from build123d import *

# Parameters (mm, degrees)
F0_R         = 5
F1_DEPTH     = 66
F2_R         = 5
F3_DEPTH     = 25
F5_DEPTH     = 11
F6_T1_DEPTH  = 14.0560753695
F6_T3_DEPTH  = 14.0560753695
F6_T5_DEPTH  = 14.0560753695
F6_T7_DEPTH  = 14.0560753695
F6_T9_DEPTH  = 14.0560753695
F6_T11_DEPTH = 14.0560753695
F6_T13_DEPTH = 17.3577997637
F6_T15_DEPTH = 17.3577997637
F6_T18_ANGLE = 298.0668340959


# Not quite as in the source:
# - a fillet or chamfer that OpenCascade refuses, or shapes differently, is made with other operations: its cross-section is extruded or revolved along the edge and cut away or added


with BuildPart() as f1:
    # F0 (on Top) → F1 (new body)
    with BuildSketch(Plane.XY):
        Circle(F0_R)
    extrude(amount=F1_DEPTH)

    # F2 (on face) → F3 (cut)
    with BuildSketch(Plane.XY.offset(66)):
        Circle(F2_R)
        Polygon((4.55, 1.8846717088), (4.55, -1.8846717088), (1.8846717088, -4.55), (-1.8846717088, -4.55), (-4.55, -1.8846717088), (-4.55, 1.8846717088), (-1.8846717088, 4.55), (1.8846717088, 4.55), align=None, mode=Mode.SUBTRACT)
    extrude(amount=-F3_DEPTH, mode=Mode.SUBTRACT)

    # F4 (on face) → F5 (cut)
    with BuildSketch(Plane(origin=(0, 0, 0), x_dir=(1, 0, 0), z_dir=(0, 0, -1))):
        with BuildLine():
            ThreePointArc((5, 0), (4.6193976626, 1.9134171618), (3.5355339059, 3.5355339059))
            Line((3.5355339059, 3.5355339059), (3.5355339059, -3.5355339059))
            ThreePointArc((3.5355339059, -3.5355339059), (4.6193976626, -1.9134171618), (5, 0))
        make_face()
        with BuildLine():
            ThreePointArc((-3.5355339059, -3.5355339059), (0, -5), (3.5355339059, -3.5355339059))
            Line((3.5355339059, -3.5355339059), (-3.5355339059, -3.5355339059))
        make_face()
    extrude(amount=-F5_DEPTH, mode=Mode.SUBTRACT)

    # F6: chamfer of 2 on 11 edges, made by hand

    # F6_s2 → F6_t1 (cut)
    with BuildSketch(Plane(origin=(-4.9695731053, 4.9695731053, 0), x_dir=(0, 0, 1), z_dir=(0.7071067812, -0.7071067812, 0))):
        Polygon((64, -4.55), (66, -2.55), (66, -4.55), align=None)
    extrude(amount=F6_T1_DEPTH, mode=Mode.SUBTRACT)

    # F6_s4 → F6_t3 (cut)
    with BuildSketch(Plane.XZ.offset(-7.0280376847)):
        Polygon((4.55, 64), (2.55, 66), (4.55, 66), align=None)
        Polygon((-4.55, 64), (-2.55, 66), (-4.55, 66), align=None)
    extrude(amount=F6_T3_DEPTH, mode=Mode.SUBTRACT)

    # F6_s6 → F6_t5 (cut)
    with BuildSketch(Plane(origin=(4.9695731053, 4.9695731053, 0), x_dir=(0, 0, 1), z_dir=(-0.7071067812, -0.7071067812, 0))):
        Polygon((64, -4.55), (66, -2.55), (66, -4.55), align=None)
    extrude(amount=F6_T5_DEPTH, mode=Mode.SUBTRACT)

    # F6_s8 → F6_t7 (cut)
    with BuildSketch(Plane.YZ.offset(-7.0280376847)):
        Polygon((-4.55, 64), (-2.55, 66), (-4.55, 66), align=None)
        Polygon((4.55, 64), (2.55, 66), (4.55, 66), align=None)
    extrude(amount=F6_T7_DEPTH, mode=Mode.SUBTRACT)

    # F6_s10 → F6_t9 (cut)
    with BuildSketch(Plane(origin=(4.9695731053, -4.9695731053, 0), x_dir=(0, 0, 1), z_dir=(-0.7071067812, 0.7071067812, 0))):
        Polygon((64, -4.55), (66, -2.55), (66, -4.55), align=None)
    extrude(amount=F6_T9_DEPTH, mode=Mode.SUBTRACT)

    # F6_s12 → F6_t11 (cut)
    with BuildSketch(Plane(origin=(-4.9695731053, -4.9695731053, 0), x_dir=(0, 0, 1), z_dir=(0.7071067812, 0.7071067812, 0))):
        Polygon((64, -4.55), (66, -2.55), (66, -4.55), align=None)
    extrude(amount=F6_T11_DEPTH, mode=Mode.SUBTRACT)

    # F6_s14 → F6_t13 (cut)
    with BuildSketch(Plane.XZ.offset(-8.6788998819)):
        Polygon((3.5355339059, 2), (1.5355339059, 0), (3.5355339059, 0), align=None)
    extrude(amount=F6_T13_DEPTH, mode=Mode.SUBTRACT)

    # F6_s16 → F6_t15 (cut)
    with BuildSketch(Plane.YZ.offset(-8.6788998819)):
        Polygon((3.5355339059, 2), (1.5355339059, 0), (3.5355339059, 0), align=None)
    extrude(amount=F6_T15_DEPTH, mode=Mode.SUBTRACT)

    # F6_s17 → F6_t18 (revolve, cut)
    with BuildSketch(Plane(origin=(0, 0, 0), x_dir=(0, 0, 1), z_dir=(0.9701544633, -0.2424877673, 0))):
        Polygon((2, -5), (0, -3), (0, -5), align=None)
    revolve(axis=Axis((0, 0, 0), (0, 0, 1)), revolution_arc=F6_T18_ANGLE, mode=Mode.SUBTRACT)


solid = f1.part
Read the model definition and answer for the solid it produces. Units are mm, in the model's axes. A direction names the side the tool comes from. Coordinates: 2 decimals unless noted, no trailing zeros. Loops run counter-clockwise (first coordinate to the right, second up) from the corner with the lowest first, then second, coordinate; pieces in that order, holes last.
Q1. Which of the six approach directions +Z, -Z, +X, -X, +Y, -Y give full straight-line access (tool end or side, diameter ignored) to faces 1 (the face through (0, 3.536, 6)), 2 (the face through (0, -4.55, 53)), 3 (the face through (3.236, -3.199, 52.661)), 4 (the face through (3.199, 3.236, 52.661)), 5 (the face through (4, 0, 11))?
Q2. Each of these flat-tipped pins is pushed along its axis until it touches: pin 1 Ø3 at (x, z) = (0, 51.5) entering from -Y; pin 2 Ø2 at (y, z) = (0.5, 6.5) entering from +X; pin 3 Ø1.1 at (y, z) = (0.5, 57.5) entering from -X. Where does it stop, or does it pass through?
Q3. Consider probe 1 along Y at (x, z) = (0, 7); probe 2 along Y at (x, z) = (1, 53.5). Determine where each line is inside the solid, lowest interval first.
Q4. The part is cut by section A-A on z = 58.5. Write down the section's boundary in (x, y), and give its area (3 significant figures).
Q5. The part is cut by section D-D on z = 28. Write down the section's boundary in (x, y).
Q6. The part is cut by section B-B on x = 0. Write down the section's boundary in (y, z).
Results below:
1. face 1: -Z, +X, -X, +Y
1. face 2: +Z, +X, -X, -Y
1. face 3: +Z, +X, -Y
1. face 4: +Z, +X, +Y
1. face 5: -Z, +X, +Y, -Y
2. pin 1: stops at y = -4.55
2. pin 2: stops at x = 3.54
2. pin 3: stops at x = -4.55
3. probe 1: y = -5 to 3.54
3. probe 2: y = -4.55 to 4.55
4. outline: (-4.55, -1.88) - (-1.88, -4.55) - (1.88, -4.55) - (4.55, -1.88) - (4.55, 1.88) - (1.88, 4.55) - (-1.88, 4.55) - (-4.55, 1.88) - close
4. area: 68.6 mm2
5. outline: circle Ø10 at (0, 0)
6. outline: (-5, 2) - (-3, 0) - (1.54, 0) - (3.54, 2) - (3.54, 11) - (5, 11) - (5, 41) - (4.55, 41) - (4.55, 64) - (2.55, 66) - (-2.55, 66) - (-4.55, 64) - (-4.55, 41) - (-5, 41) - close
